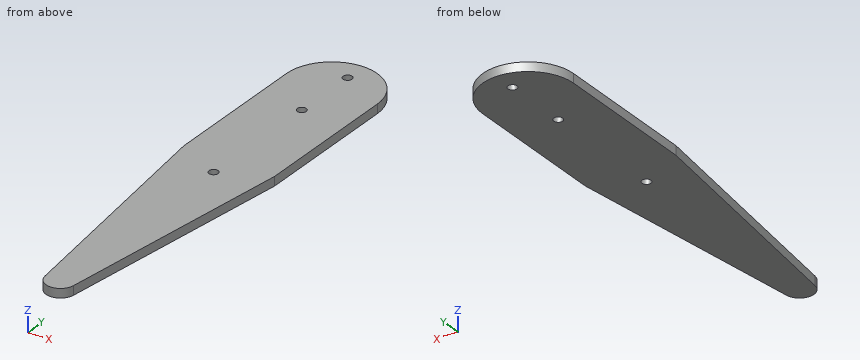
```python
from build123d import *

# Parameters (mm, degrees)
SKETCH1_R           = 1.5
BOSS_EXTRUDE1_DEPTH = 3


with BuildPart() as part:
    # Sketch1 → Boss-Extrude1 (new body)
    with BuildSketch(Plane.XY):
        with BuildLine():
            Line((-5, 44.75), (-5, -4.25))
            Line((-5, -4.25), (5.287636044, -85.486762889))
            ThreePointArc((5.287636044, -85.486762889), (10, -89.64), (14.712363956, -85.486762889))
            Line((14.712363956, -85.486762889), (25, -4.25))
            Line((25, -4.25), (25, 44.75))
            ThreePointArc((25, 44.75), (10, 59.75), (-5, 44.75))
        make_face()
        with Locations((10, 30.36)):
            Circle(SKETCH1_R, mode=Mode.SUBTRACT)
        with Locations((10, 52.25)):
            Circle(SKETCH1_R, mode=Mode.SUBTRACT)
        with Locations((10, -11.75)):
            Circle(SKETCH1_R, mode=Mode.SUBTRACT)
    extrude(amount=BOSS_EXTRUDE1_DEPTH)


solid = part.part
```
Can you work these out from the model? Positions are in its coordinate system, mm. Give positions to 0.01 mm unless a question says otherwise; leave off trailing zeros. Loops run counter-clockwise (first coordinate to the right, second up) from the corner with the lowest first, then second, coordinate; pieces in that order, holes last. Notation, with made-up numbers: M 50,7 L 107,7 A12 cw 107,20 Z; hole C 40,-22 d5. An arc over 180 degrees is marked long. Use CSV: the item, a comma, the result in double quotes. Start each with the question number.
1. Imagine slicing it at D-D, the plane y = -11.75. Write out the boundary of the cut face in (x, z), plus the area to 3 significant figures.
2. Imagine slicing it at B-B, the plane y = 30.36. Write out the boundary of the cut face in (x, z), plus the area to 3 significant figures.
3. For P1, Ø1.5, axis at x = 20, z = 2.5, coming from the +Y side; P2, Ø1, axis at x = 20, y = -61.5, coming from the +Z side, each with a flat end and sliding along its axis, tell me the tip position at first contact or that it passes through.
4. If I drill on L1, parallel to Y at x = 10, z = 1.8; L2, parallel to Y at x = 11, z = 1.7; L3, parallel to X at y = -10.5, z = 0.4, over which ranges is the centre line in solid material (lowest first)?
5. Imagine slicing it at C-C, the plane z = 2. Write out the boundary of the cut face in (x, y), plus the area to 3 significant figures.
6. Imagine slicing it at A-A, the plane x = 10. Write out the boundary of the cut face in (y, z), plus the area to 3 significant figures.
Response values:
1,outline,"M -4.05,0 L 8.5,0 L 8.5,3 L -4.05,3 Z; M 11.5,0 L 24.05,0 L 24.05,3 L 11.5,3 Z"
1,area,"75.3 mm^2"
2,outline,"M -5,0 L 8.5,0 L 8.5,3 L -5,3 Z; M 11.5,0 L 25,0 L 25,3 L 11.5,3 Z"
2,area,"81.0 mm^2"
3,P1,"y = 56.56"
3,P2,"through"
4,L1,"-89.64 to -13.25, -10.25 to 28.86, 31.86 to 50.75, 53.75 to 59.75"
4,L2,"-89.53 to -12.87, -10.63 to 29.24, 31.48 to 51.13, 53.37 to 59.72"
4,L3,"-4.21 to 9.17, 10.83 to 24.21"
5,outline,"M -5,-4.25 L 5.29,-85.49 A4.75 ccw 14.71,-85.49 L 25,-4.25 L 25,44.75 A15 ccw -5,44.75 Z; hole C 10,-11.75 d3; hole C 10,30.36 d3; hole C 10,52.25 d3"
5,area,"3,430 mm^2"
6,outline,"M -89.64,0 L -13.25,0 L -13.25,3 L -89.64,3 Z; M -10.25,0 L 28.86,0 L 28.86,3 L -10.25,3 Z; M 31.86,0 L 50.75,0 L 50.75,3 L 31.86,3 Z; M 53.75,0 L 59.75,0 L 59.75,3 L 53.75,3 Z"
6,area,"421 mm^2"
